```python
from build123d import *

# Parameters (mm, degrees)
SKETCH1_R           = 75
SKETCH1_R_2         = 4
SKETCH1_R_3         = 14.75
SKETCH1_R_4         = 1.75
BOSS_EXTRUDE1_DEPTH = 12
SKETCH2_W           = 20
SKETCH2_H           = 8
SKETCH2_W_2         = 8
SKETCH2_H_2         = 10
SKETCH2_W_3         = 7
SKETCH2_H_3         = 4
CUT_EXTRUDE1_DEPTH  = 8
CUT_EXTRUDE2_REACH  = 108.743
SKETCH3_R           = 2.65
SKETCH4_R           = 2.121320344
SKETCH4_R_2         = 2
CUT_EXTRUDE3_DEPTH  = 8
CUT_EXTRUDE4_REACH  = 108.743
SKETCH5_R           = 1.6


with BuildPart() as part:
    # Sketch1 → Boss-Extrude1 (new body)
    with BuildSketch(Plane(origin=(0, 0, 0), x_dir=(0, 0, -1), z_dir=(1, 0, 0))):
        Circle(SKETCH1_R)
        with Locations((0, 50)):
            Circle(SKETCH1_R_2, mode=Mode.SUBTRACT)
        with Locations((43.301270189, -25)):
            Circle(SKETCH1_R_2, mode=Mode.SUBTRACT)
        with Locations((-43.301270189, -25)):
            Circle(SKETCH1_R_2, mode=Mode.SUBTRACT)
        with Locations((26.1, 0)):
            Circle(SKETCH1_R_3, mode=Mode.SUBTRACT)
        with Locations(Location((-26.1, 0, 0), (0, 0, 180))):
            Circle(SKETCH1_R_3, mode=Mode.SUBTRACT)
        with Locations((39.596900686, 13.496900686)):
            Circle(SKETCH1_R_4, mode=Mode.SUBTRACT)
        with Locations((39.596900686, -13.496900686)):
            Circle(SKETCH1_R_4, mode=Mode.SUBTRACT)
        with Locations((12.603099314, -13.496900686)):
            Circle(SKETCH1_R_4, mode=Mode.SUBTRACT)
        with Locations((12.603099314, 13.496900686)):
            Circle(SKETCH1_R_4, mode=Mode.SUBTRACT)
        with Locations(Location((-39.596900686, -13.496900686, 0), (0, 0, 180))):
            Circle(SKETCH1_R_4, mode=Mode.SUBTRACT)
        with Locations(Location((-12.603099314, -13.496900686, 0), (0, 0, 180))):
            Circle(SKETCH1_R_4, mode=Mode.SUBTRACT)
        with Locations(Location((-12.603099314, 13.496900686, 0), (0, 0, 180))):
            Circle(SKETCH1_R_4, mode=Mode.SUBTRACT)
        with Locations(Location((-39.596900686, 13.496900686, 0), (0, 0, 180))):
            Circle(SKETCH1_R_4, mode=Mode.SUBTRACT)
    extrude(amount=BOSS_EXTRUDE1_DEPTH)

    # Sketch2 → Cut-Extrude1 (cut)
    with BuildSketch(Plane(origin=(12, 0, 0), x_dir=(0, 0, -1), z_dir=(1, 0, 0))):
        with Locations((20, -31.5)):
            Rectangle(SKETCH2_W, SKETCH2_H)
        with Locations((-20, -31.5)):
            Rectangle(SKETCH2_W, SKETCH2_H)
        with Locations((-20, 31.5)):
            Rectangle(SKETCH2_W, SKETCH2_H)
        with Locations((20, 31.5)):
            Rectangle(SKETCH2_W, SKETCH2_H)
        with Locations((0, -22.5)):
            Rectangle(SKETCH2_W_2, SKETCH2_H_2)
        with Locations((0, 22.5)):
            Rectangle(SKETCH2_W_2, SKETCH2_H_2)
        with Locations((-9, -65)):
            Rectangle(SKETCH2_W_3, SKETCH2_H_3)
        with Locations((9, -65)):
            Rectangle(SKETCH2_W_3, SKETCH2_H_3)
    extrude(amount=-CUT_EXTRUDE1_DEPTH, mode=Mode.SUBTRACT)

    # Sketch3 → Cut-Extrude2 (cut, up to next)
    with BuildSketch(Plane.ZY, mode=Mode.PRIVATE) as cut_extrude2_sk1:
        with Locations((-70, 0)):
            Circle(SKETCH3_R)
    cut_extrude2_tool1 = extrude(cut_extrude2_sk1.sketch, amount=-CUT_EXTRUDE2_REACH, mode=Mode.PRIVATE) & part.part
    # Sketch3 → Cut-Extrude2 (cut, up to next)
    with BuildSketch(Plane.ZY, mode=Mode.PRIVATE) as cut_extrude2_sk2:
        with Locations((-35, 60.621778265)):
            Circle(SKETCH3_R)
    cut_extrude2_tool2 = extrude(cut_extrude2_sk2.sketch, amount=-CUT_EXTRUDE2_REACH, mode=Mode.PRIVATE) & part.part
    # Sketch3 → Cut-Extrude2 (cut, up to next)
    with BuildSketch(Plane.ZY, mode=Mode.PRIVATE) as cut_extrude2_sk3:
        with Locations((35, 60.621778265)):
            Circle(SKETCH3_R)
    cut_extrude2_tool3 = extrude(cut_extrude2_sk3.sketch, amount=-CUT_EXTRUDE2_REACH, mode=Mode.PRIVATE) & part.part
    # Sketch3 → Cut-Extrude2 (cut, up to next)
    with BuildSketch(Plane.ZY, mode=Mode.PRIVATE) as cut_extrude2_sk4:
        with Locations((70, 0)):
            Circle(SKETCH3_R)
    cut_extrude2_tool4 = extrude(cut_extrude2_sk4.sketch, amount=-CUT_EXTRUDE2_REACH, mode=Mode.PRIVATE) & part.part
    # Sketch3 → Cut-Extrude2 (cut, up to next)
    with BuildSketch(Plane.ZY, mode=Mode.PRIVATE) as cut_extrude2_sk5:
        with Locations((35, -60.621778265)):
            Circle(SKETCH3_R)
    cut_extrude2_tool5 = extrude(cut_extrude2_sk5.sketch, amount=-CUT_EXTRUDE2_REACH, mode=Mode.PRIVATE) & part.part
    # Sketch3 → Cut-Extrude2 (cut, up to next)
    with BuildSketch(Plane.ZY, mode=Mode.PRIVATE) as cut_extrude2_sk6:
        with Locations((-35, -60.621778265)):
            Circle(SKETCH3_R)
    cut_extrude2_tool6 = extrude(cut_extrude2_sk6.sketch, amount=-CUT_EXTRUDE2_REACH, mode=Mode.PRIVATE) & part.part
    add(cut_extrude2_tool1.solids().sort_by_distance((0, 0, -70))[0], mode=Mode.SUBTRACT)
    add(cut_extrude2_tool2.solids().sort_by_distance((0, 60.621778, -35))[0], mode=Mode.SUBTRACT)
    add(cut_extrude2_tool3.solids().sort_by_distance((0, 60.621778, 35))[0], mode=Mode.SUBTRACT)
    add(cut_extrude2_tool4.solids().sort_by_distance((0, 0, 70))[0], mode=Mode.SUBTRACT)
    add(cut_extrude2_tool5.solids().sort_by_distance((0, -60.621778, 35))[0], mode=Mode.SUBTRACT)
    add(cut_extrude2_tool6.solids().sort_by_distance((0, -60.621778, -35))[0], mode=Mode.SUBTRACT)

    # Sketch4 → Cut-Extrude3 (cut)
    with BuildSketch(Plane(origin=(12, 0, 0), x_dir=(0, 0, -1), z_dir=(1, 0, 0))):
        with Locations((-10, -35.5)):
            Circle(SKETCH4_R)
        with Locations((-10, -27.5)):
            Circle(SKETCH4_R)
        with Locations((-30, -27.5)):
            Circle(SKETCH4_R)
        with Locations((-30, -35.5)):
            Circle(SKETCH4_R)
        with Locations((12.5, -65)):
            Circle(SKETCH4_R_2)
        with Locations((5.5, -65)):
            Circle(SKETCH4_R_2)
        with Locations((-5.5, -65)):
            Circle(SKETCH4_R_2)
        with Locations((-12.5, -65)):
            Circle(SKETCH4_R_2)
        with Locations((10, -35.5)):
            Circle(SKETCH4_R)
        with Locations((10, -27.5)):
            Circle(SKETCH4_R)
        with Locations((30, -27.5)):
            Circle(SKETCH4_R)
        with Locations((30, -35.5)):
            Circle(SKETCH4_R)
        with Locations((4, -27.5)):
            Circle(SKETCH4_R)
        with Locations((-4, -27.5)):
            Circle(SKETCH4_R)
        with Locations((-4, -17.5)):
            Circle(SKETCH4_R)
        with Locations((4, -17.5)):
            Circle(SKETCH4_R)
        with Locations((4, 27.5)):
            Circle(SKETCH4_R)
        with Locations((-4, 27.5)):
            Circle(SKETCH4_R)
        with Locations((-4, 17.5)):
            Circle(SKETCH4_R)
        with Locations((4, 17.5)):
            Circle(SKETCH4_R)
        with Locations((10, 27.5)):
            Circle(SKETCH4_R)
        with Locations((10, 35.5)):
            Circle(SKETCH4_R)
        with Locations((30, 35.5)):
            Circle(SKETCH4_R)
        with Locations((30, 27.5)):
            Circle(SKETCH4_R)
        with Locations((-10, 35.5)):
            Circle(SKETCH4_R)
        with Locations((-10, 27.5)):
            Circle(SKETCH4_R)
        with Locations((-30, 27.5)):
            Circle(SKETCH4_R)
        with Locations((-30, 35.5)):
            Circle(SKETCH4_R)
    extrude(amount=-CUT_EXTRUDE3_DEPTH, mode=Mode.SUBTRACT)

    # Sketch5 → Cut-Extrude4 (cut, up to next)
    with BuildSketch(Plane.ZY, mode=Mode.PRIVATE) as cut_extrude4_sk1:
        with Locations((25.403411844, -44)):
            Circle(SKETCH5_R)
    cut_extrude4_tool1 = extrude(cut_extrude4_sk1.sketch, amount=-CUT_EXTRUDE4_REACH, mode=Mode.PRIVATE) & part.part
    # Sketch5 → Cut-Extrude4 (cut, up to next)
    with BuildSketch(Plane.ZY, mode=Mode.PRIVATE) as cut_extrude4_sk2:
        with Locations((-25.403411844, 44)):
            Circle(SKETCH5_R)
    cut_extrude4_tool2 = extrude(cut_extrude4_sk2.sketch, amount=-CUT_EXTRUDE4_REACH, mode=Mode.PRIVATE) & part.part
    add(cut_extrude4_tool1.solids().sort_by_distance((0, -44, 25.403412))[0], mode=Mode.SUBTRACT)
    add(cut_extrude4_tool2.solids().sort_by_distance((0, 44, -25.403412))[0], mode=Mode.SUBTRACT)


solid = part.part
```
Geometry: final body of the model. Coordinates: model frame, mm. A direction names the side the tool comes from. Round coordinates to 2 decimals unless told otherwise and drop trailing zeros. Loops run counter-clockwise (first coordinate to the right, second up) from the corner with the lowest first, then second, coordinate; pieces in that order, holes last. Notation, with made-up numbers: (11.25, 71) -> (69.25, 71) arc R13 ccw to (69.25, 82) -> close; hole circle Ø6 at (3, -35.75). An arc over 180 degrees is marked (long way). Use one line per item in the form item = value.
Item 1: Material intervals for probe 1 along Y at (x, z) = (6.5, 29); probe 2 along Y at (x, z) = (5.5, -27.5); probe 3 along Y at (x, z) = (11, 9.5), sorted ascending.
Evaluation:
probe_1 = -69.17 to -37.37, -25.63 to -14.46, 14.46 to 25.63, 37.37 to 69.17
probe_2 = -69.78 to -35.5, -27.5 to -14.68, 14.68 to 27.5, 35.5 to 69.78
probe_3 = -74.4 to -67, -63 to -37.56, -33.44 to -29.56, -25.44 to 25.44, 29.56 to 33.44, 37.56 to 74.4
Item 2: Access query for faces 1 (the cylindrical face through (5.92, -12.83, 14.22)), 2 (the cylindrical face through (8.06, 37.05, -8.55)). Directions: +Z, -Z, +X, -X, +Y, -Y. A direction counts if a zero-diameter tool reaches every point of the face in a straight line with its end or side. Return the directions, or none.
Evaluation:
face_1 = +X, -X
face_2 = +X
Item 3: Cut plane B-B on x = 1.75. Give the number of separate pieces and of enclosed holes in the cut face, then the cut area to 3 significant figures.
Evaluation:
separate_pieces = 1
enclosed_holes = 21
area = 15,900 mm2
Item 4: Cut plane A-A on z = 0. Output: boundary loops of the cut face in (x, y).
Evaluation:
outline = (0, -75) -> (12, -75) -> (12, -27.5) -> (4, -27.5) -> (4, -17.5) -> (12, -17.5) -> (12, 17.5) -> (4, 17.5) -> (4, 27.5) -> (12, 27.5) -> (12, 46) -> (0, 46) -> close; (0, 54) -> (12, 54) -> (12, 75) -> (0, 75) -> close
Item 5: Cut plane C-C on y = -65. Output: boundary loops of the cut face in (x, z).
Evaluation:
outline = (0, -37.42) -> (12, -37.42) -> (12, -14.5) -> (4, -14.5) -> (4, -3.5) -> (12, -3.5) -> (12, 3.5) -> (4, 3.5) -> (4, 14.5) -> (12, 14.5) -> (12, 37.42) -> (0, 37.42) -> close
Item 6: Cut plane D-D on z = 17.5. Output: boundary loops of the cut face in (x, y), then the cut area to 3 significant figures.
Evaluation:
outline = (0, -72.93) -> (12, -72.93) -> (12, -35.5) -> (4, -35.5) -> (4, -27.5) -> (12, -27.5) -> (12, -11.98) -> (0, -11.98) -> close; (0, 11.98) -> (12, 11.98) -> (12, 27.5) -> (4, 27.5) -> (4, 35.5) -> (12, 35.5) -> (12, 72.93) -> (0, 72.93) -> close
area = 1,330 mm2
Item 7: Contact query for flat-ended pins moving along their axis: pin 1 Ø2 at (x, z) = (4, 47) entering from -Y; pin 2 Ø4 at (x, y) = (7, 32) entering from +Z; pin 3 Ø2 at (x, z) = (6.5, -9) entering from +Y. Output: stop coordinate, or through.
Evaluation:
pin_1 = -59.24
pin_2 = 68.74
pin_3 = 74.57
